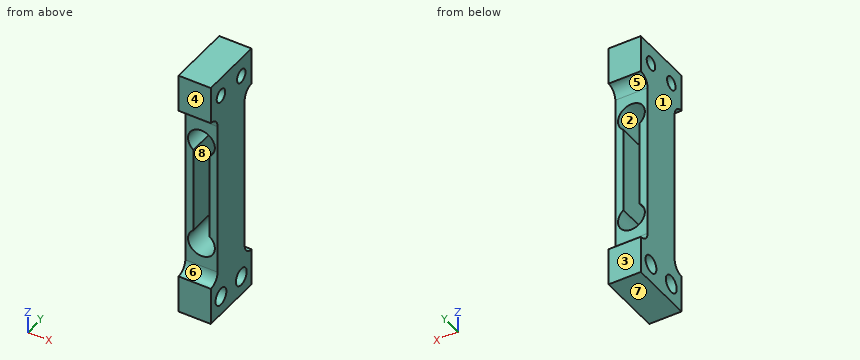
```python
from build123d import *

# Parameters (mm, degrees)
SKETCH1_W                 = 47
SKETCH1_H                 = 12
BOSS_EXTRUDE1_DEPTH       = 6
CUT_EXTRUDE2_DEPTH        = 25.984995497
SKETCH4_R                 = 1.6
CUT_EXTRUDE3_DEPTH        = 25.984995497
M3X0_5_TAPPED_HOLE1_D     = 2.5
M3X0_5_TAPPED_HOLE1_DEPTH = 7.5
M3X0_5_TAPPED_HOLE1_TIP   = 0.751075774
CUT_EXTRUDE4_DEPTH        = 27.234519245


with BuildPart() as part:
    # Sketch1 → Boss-Extrude1 (new body)
    with BuildSketch(Plane(origin=(0, 0, 0), x_dir=(0, 0, -1), z_dir=(1, 0, 0))):
        Rectangle(SKETCH1_W, SKETCH1_H)
    extrude(amount=BOSS_EXTRUDE1_DEPTH)

    # Sketch3 → Cut-Extrude2 (cut, through all)
    with BuildSketch(Plane(origin=(6, 0, 0), x_dir=(0, 0, -1), z_dir=(1, 0, 0))):
        with BuildLine():
            Line((16.5, 6), (-16.5, 6))
            ThreePointArc((-16.5, 6), (-15.914213562, 4.585786438), (-14.5, 4))
            Line((-14.5, 4), (14.5, 4))
            ThreePointArc((14.5, 4), (15.914213562, 4.585786438), (16.5, 6))
        make_face()
        with BuildLine():
            Line((-14.5, -4), (14.5, -4))
            ThreePointArc((14.5, -4), (15.914213562, -4.585786438), (16.5, -6))
            Line((16.5, -6), (-16.5, -6))
            ThreePointArc((-16.5, -6), (-15.914213562, -4.585786438), (-14.5, -4))
        make_face()
    extrude(amount=-CUT_EXTRUDE2_DEPTH, mode=Mode.SUBTRACT)

    # Sketch4 → Cut-Extrude3 (cut, through all)
    with BuildSketch(Plane(origin=(6, 0, 0), x_dir=(0, 0, -1), z_dir=(1, 0, 0))):
        with Locations((20, 3)):
            Circle(SKETCH4_R)
        with Locations((20, -3)):
            Circle(SKETCH4_R)
    extrude(amount=-CUT_EXTRUDE3_DEPTH, mode=Mode.SUBTRACT)

    # M3x0.5 Tapped Hole1
    with Locations(Plane(origin=(6, 0, 0), x_dir=(0, 0, -1), z_dir=(1, 0, 0))):
        with Locations((-20, 3), (-20, -3)):
            Hole(M3X0_5_TAPPED_HOLE1_D / 2, depth=M3X0_5_TAPPED_HOLE1_DEPTH)
            with Locations((0, 0, -(M3X0_5_TAPPED_HOLE1_DEPTH + M3X0_5_TAPPED_HOLE1_TIP / 2))):  # 118° drill point
                Cone(0, M3X0_5_TAPPED_HOLE1_D / 2, M3X0_5_TAPPED_HOLE1_TIP, mode=Mode.SUBTRACT)

    # Sketch8 → Cut-Extrude4 (cut, through all)
    with BuildSketch(Plane.XZ.offset(4)):
        with BuildLine():
            Line((4.5, 8), (4.5, -8))
            ThreePointArc((4.5, -8), (3, -12.5), (1.5, -8))
            Line((1.5, -8), (1.5, 8))
            ThreePointArc((1.5, 8), (3, 12.5), (4.5, 8))
        make_face()
    extrude(amount=-CUT_EXTRUDE4_DEPTH, mode=Mode.SUBTRACT)


solid = part.part
```
CAD build for the part. Positions are in the model's coordinates, mm. Face numbers are marked on the shaded views. A direction names the side the tool comes from. Round coordinates to 2 decimals unless told otherwise and drop trailing zeros. Loops run counter-clockwise (first coordinate to the right, second up) from the corner with the lowest first, then second, coordinate; pieces in that order, holes last. Notation, with made-up numbers: M 32,-11.5 L 85,-11.5 A13 cw 85,1.5 Z; hole C 71.5,69.5 d1. An arc over 180 degrees is marked long. Use a Markdown table: item, result. Add a question column.
(1) Which spindle directions (+Z, -Z, +X, -X, +Y, -Y) get a long thin tool onto all of the face, cutting with end or side? Do the marked faces 4, 5, 6, 7 and 8. Say none if no direction does.
(2) Pull direction X, two halves, no side cores. Call the marked faces 1, 2 and 3: +X half, -X half, draft (parallel to the pull), parting line (faces both ways), or undercut.
(3) Cut at A-A (y = -3). Give the cut face in (x, z), and give its area (3 significant figures).
(4) Flat gauge pins, fed straight in: pin 1 (4 mm diameter, centred on y = -1, z = -4, fed in from -X); pin 2 (1.8 mm diameter, centred on x = 2, z = 3.5, fed in from -Y). Where does each tip first touch, or does it go through?
(5) Cut at B-B (z = 20). Give the cut face in (x, y), and give its area (3 significant figures).
(6) Cut at D-D (z = -7). Give the cut face in (x, y).
(7) Cut at C-C (x = 3). Give the cut face in (y, z), and give its area (3 significant figures).
(8) Drill centre lines: line 1 (Y direction, x = 2.65, z = 20); line 2 (X direction, y = -2, z = -10); line 3 (X direction, y = -3.5, z = -7.5). Where is each one in solid material? Low to high.
Geometry says:
| question | item | result |
|---|---|---|
| 1 | face 4 | +Z, -Z, +X, -X, -Y |
| 1 | face 5 | +X, -X, +Y |
| 1 | face 6 | +X, -X, -Y |
| 1 | face 7 | -Z, +X, -X, +Y, -Y |
| 1 | face 8 | +Y, -Y |
| 2 | face 1 | -X half |
| 2 | face 2 | undercut |
| 2 | face 3 | draft |
| 3 | outline | M 0,-23.5 L 6,-23.5 L 6,-21.6 L 0,-21.6 Z; M 0,-18.4 L 6,-18.4 L 6,18.75 L 0,18.75 Z; M 0,21.25 L 6,21.25 L 6,23.5 L 0,23.5 Z; hole M 1.5,-8 A2.5 ccw long 4.5,-8 L 4.5,8 A2.5 ccw long 1.5,8 Z |
| 3 | area | 163 mm² |
| 4 | pin 1 | stops at x = 0 |
| 4 | pin 2 | stops at y = -4 |
| 5 | outline | M 0,-6 L 6,-6 L 6,-4.25 L 0,-4.25 Z; M 0,-1.75 L 6,-1.75 L 6,1.75 L 0,1.75 Z; M 0,4.25 L 6,4.25 L 6,6 L 0,6 Z |
| 5 | area | 42.0 mm² |
| 6 | outline | M 0,-4 L 1.5,-4 L 1.5,4 L 0,4 Z; M 4.5,-4 L 6,-4 L 6,4 L 4.5,4 Z |
| 7 | outline | M -6,-23.5 L 6,-23.5 L 6,-16.5 A2 cw 4,-14.5 L 4,-12.5 L -4,-12.5 L -4,-14.5 A2 cw -6,-16.5 Z; M -6,16.5 A2 cw -4,14.5 L -4,12.5 L 4,12.5 L 4,14.5 A2 cw 6,16.5 L 6,23.5 L -6,23.5 Z; hole C -3,-20 d3.2; hole C -3,20 d2.5; hole C 3,-20 d3.2; hole C 3,20 d2.5 |
| 7 | area | 210 mm² |
| 8 | line 1 | y = -6 to -4.25, -1.75 to 1.75, 4.25 to 6 |
| 8 | line 2 | x = 0 to 0.5, 5.5 to 6 |
| 8 | line 3 | x = 0 to 1.5, 4.5 to 6 |
